```python
from build123d import *

# Parameters (mm, degrees)
CROQUIS1_R              = 1.5
SALIENTE_EXTRUIR1_DEPTH = 2.6


with BuildPart() as part:
    # Croquis1 → Saliente-Extruir1 (new body)
    with BuildSketch(Plane(origin=(0, 0, 0), x_dir=(1, 0, 0), z_dir=(0, 1, 0))):
        with BuildLine():
            ThreePointArc((10.705140116, 13.624644249), (0, 17.327173913), (-10.705140116, 13.624644249))
            ThreePointArc((-10.705140116, 13.624644249), (-16.602529664, 14.332314029), (-15.894859884, 20.229703577))
            ThreePointArc((-15.894859884, 20.229703577), (0, 25.727173913), (15.894859884, 20.229703577))
            ThreePointArc((15.894859884, 20.229703577), (16.602529664, 14.332314029), (10.705140116, 13.624644249))
        make_face()
        with Locations(Location((13.3, 16.927173913, 0), (0, 0, 270))):
            Circle(CROQUIS1_R, mode=Mode.SUBTRACT)
        with Locations(Location((-13.3, 16.927173913, 0), (0, 0, 270))):
            Circle(CROQUIS1_R, mode=Mode.SUBTRACT)
    extrude(amount=SALIENTE_EXTRUIR1_DEPTH)


solid = part.part
```
Verification items for the finished model (mm, model axes). Round coordinates to 2 decimals unless told otherwise and drop trailing zeros. Order: outer loops, then holes, each group sorted by start corner. A loop starts at its lowest first (then second) coordinate and runs counter-clockwise, first axis right, second up. Notation, with made-up numbers: (73.25, 87) - (91.25, 87) arc R5 cw to (91.25, 92) - close; hole circle Ø2 at (63, 62). An arc over 180 degrees is marked (long way). Use CSV: the item, a comma, the result in double quotes.
(1) Section check C-C on x = 13.3. Record the boundary of the cut face in (y, z).
Entries:
outline,"(0, -22.02) - (2.6, -22.02) - (2.6, -18.43) - (0, -18.43) - close; (0, -15.43) - (2.6, -15.43) - (2.6, -12.73) - (0, -12.73) - close"
(2) Section check A-A on y = 0.8. Record the boundary of the cut face in (x, z).
Entries:
outline,"(-15.89, -20.23) arc R25.73 ccw to (15.89, -20.23) arc R4.2 ccw to (10.71, -13.62) arc R17.33 cw to (-10.71, -13.62) arc R4.2 ccw to start; hole circle Ø3 at (-13.3, -16.93); hole circle Ø3 at (13.3, -16.93)"
(3) Section check B-B on z = -14.25. Record the boundary of the cut face in (x, y).
Entries:
outline,"(-16.54, 0) - (-9.86, 0) - (-9.86, 2.6) - (-16.54, 2.6) - close; (9.86, 0) - (16.54, 0) - (16.54, 2.6) - (9.86, 2.6) - close"
(4) Gauge pin test, flat end, axial feed: pin 1 Ø3.5 at (x, z) = (-13.3, -16.93) entering from +Y. Record the tip position at first contact, or that the pin passes through.
Entries:
pin 1,"y = 2.6"
(5) Mould release check, pull along X, two halves, no side actions. Record for faces 1 (the face through (0.162, 1.282, -17.326)), 2 (the face through (0, 0, -19)), 3 (the face through (-0.24, 1.282, -25.726)): released by +X, released by -X, zero draft, split by the parting line, or undercut.
Entries:
face 1,"undercut"
face 2,"zero draft"
face 3,"split by the parting line"
(6) Thickness scan on probe 1 along X at (y, z) = (1.4, -18.25); probe 2 along X at (y, z) = (0.95, -17.5); probe 3 along X at (y, z) = (2.55, -15). Record the ranges inside material, lowest first. Write a range as from..to.
Entries:
probe 1,"-17.29..-14.01, -12.59..12.59, 14.01..17.29"
probe 2,"-17.46..-14.69, -11.91..11.91, 14.69..17.46"
probe 3,"-17.03..-8.67, 8.67..17.03"
(7) Section check D-D on z = -16.5. Record the boundary of the cut face in (x, y).
Entries:
outline,"(-17.48, 0) - (-14.74, 0) - (-14.74, 2.6) - (-17.48, 2.6) - close; (-11.86, 0) - (-5.29, 0) - (-5.29, 2.6) - (-11.86, 2.6) - close; (5.29, 0) - (11.86, 0) - (11.86, 2.6) - (5.29, 2.6) - close; (14.74, 0) - (17.48, 0) - (17.48, 2.6) - (14.74, 2.6) - close"
